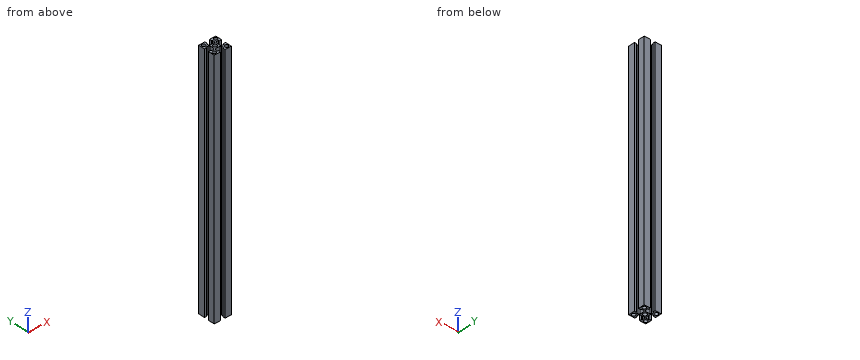
```python
from build123d import *

# Parameters (mm, degrees)
SKETCH_1_R      = 2
SKETCH_1_R_2    = 2.15
EXTRUDE_1_DEPTH = 145


with BuildPart() as part:
    # 스케치1 → 보스-돌출1 (new, symmetric)
    with BuildSketch(Plane.XY):
        Polygon((-10, -10), (-2.65, -10), (-2.65, -7.35), (-3.65, -7.35), (-3.65, -4.639949494), (-2.510050506, -3.5), (0, -3.5), (2.510050506, -3.5), (3.65, -4.639949494), (3.65, -7.35), (2.65, -7.35), (2.65, -10), (10, -10), (10, -2.65), (7.35, -2.65), (7.35, -3.65), (4.639949494, -3.65), (3.5, -2.510050506), (3.5, 0), (3.5, 2.510050506), (4.639949494, 3.65), (7.35, 3.65), (7.35, 2.65), (10, 2.65), (10, 10), (2.65, 10), (2.65, 7.35), (3.65, 7.35), (3.65, 4.639949494), (2.510050506, 3.5), (0, 3.5), (-2.510050506, 3.5), (-3.65, 4.639949494), (-3.65, 7.35), (-2.65, 7.35), (-2.65, 10), (-10, 10), (-10, 2.65), (-7.35, 2.65), (-7.35, 3.65), (-4.639949494, 3.65), (-3.5, 2.510050506), (-3.5, 0), (-3.5, -2.510050506), (-4.639949494, -3.65), (-7.35, -3.65), (-7.35, -2.65), (-10, -2.65), align=None)
        with Locations((-7, 7)):
            Circle(SKETCH_1_R, mode=Mode.SUBTRACT)
        Circle(SKETCH_1_R_2, mode=Mode.SUBTRACT)
        with Locations((7, 7)):
            Circle(SKETCH_1_R, mode=Mode.SUBTRACT)
        with Locations((-7, -7)):
            Circle(SKETCH_1_R, mode=Mode.SUBTRACT)
        with Locations((7, -7)):
            Circle(SKETCH_1_R, mode=Mode.SUBTRACT)
    extrude(amount=EXTRUDE_1_DEPTH, both=True)


solid = part.part
```
The model under review builds one solid part; all positions refer to its coordinate system, in mm. Give positions to 0.01 mm unless a question says otherwise; leave off trailing zeros. Answer in a Markdown table with one row per item.
1) For L1, parallel to Y at x = -7, z = -9; L2, parallel to Y at x = 4.5, z = 88.5; L3, parallel to Y at x = -6.5, z = -63.5, list the stretches that pass through material, from the lowest coordinate up. Write a range as [from, to].
Worked answers:
| item | result |
|---|---|
| L1 | [-10, -9], [-5, -3.65], [3.65, 5], [9, 10] |
| L2 | [-10, -3.51], [3.51, 10] |
| L3 | [-10, -8.94], [-5.06, -3.65], [3.65, 5.06], [8.94, 10] |
2) Clearance check with flat-ended pins moving along their axes: P1, Ø8, axis at x = 1, y = 0.5, coming from the +Z side; P2, Ø2, axis at x = 6.5, y = 6.5, coming from the -Z side; P3, Ø1.5, axis at x = 0, z = 10.5, coming from the -Y side. State where each tip first meets the part, or that it passes through.
Worked answers:
| item | result |
|---|---|
| P1 | z = 145 |
| P2 | through |
| P3 | y = -3.5 |
3) Add section A-A on z = -4. Count the separate pieces of the cut face and the enclosed holes in it, plus the area to 3 significant figures.
Worked answers:
| item | result |
|---|---|
| separate pieces | 1 |
| enclosed holes | 5 |
| area | 172 mm² |
